Verification items for the finished model (mm, model axes). Face numbers are marked on the shaded views. A direction names the side the tool comes from. Round coordinates to 2 decimals unless told otherwise and drop trailing zeros. Write each loop counter-clockwise with the first axis right and the second up, starting at its lowest first coordinate (ties: lowest second). Pieces come first, ordered by that corner, then holes. Notation, with made-up numbers: M -27,43.5 L 22,43.5 A30 ccw 22,66.5 Z; hole C 8.25,89 d9. An arc over 180 degrees is marked long. Answer in a Markdown table with one row per item. Add a question column.
1. Go/stop test with flat-tipped pins: pin 1 Ø3 at (x, y) = (4, 75.5) entering from +Z; pin 2 Ø4 at (y, z) = (25.4, 12.7) entering from +X; pin 3 Ø4 at (x, z) = (5.5, 111) entering from +Y; pin 4 Ø4 at (x, y) = (3, 86) entering from -Z. Record where each tip stops, or that it passes through.
2. Sectioned sample at C-C on y = 95.25. Record the cut outline in (x, z).
3. Set-up check for the marked faces 1, 2 and 3: record each of +Z, -Z, +X, -X, +Y, -Y from which the full face is reachable in a straight line by a thin tool's end or side.
4. Sectioned sample at B-B on x = 2. Record the cut outline in (y, z), plus the area to 3 significant figures.
5. Sectioned sample at A-A on z = 31.75. Record the cut outline in (x, y), plus the area to 3 significant figures.
6. Material ranges on probe 1 along Y at (x, z) = (3.5, 25.4); probe 2 along Y at (x, z) = (8.25, 31.75); probe 3 along Z at (x, y) = (10, 80.5), recorded low to high.
7. Sectioned sample at D-D on z = 88.9. Record the cut outline in (x, y), plus the area to 3 significant figures.
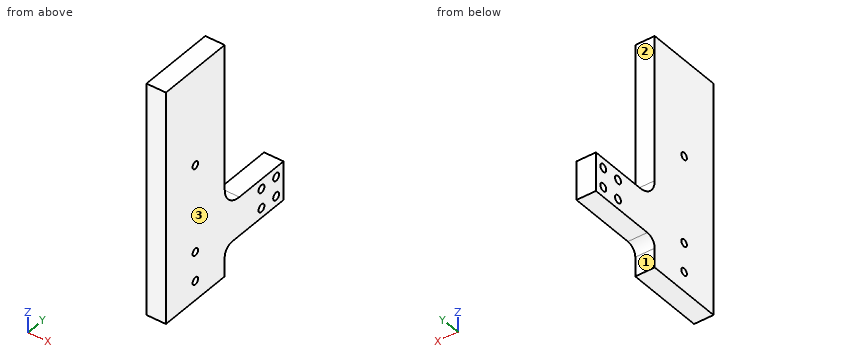
```python
from build123d import *

# Parameters (mm, degrees)
SKETCH1_R              = 2.38125
BOSS_EXTRUDE1_DEPTH    = 12.7
F_10_CLEARANCE_HOLE1_D = 5.1054
FILLET1_R              = 12.7
FILLET2_R              = 6.35


with BuildPart() as part:
    # Sketch1 → Boss-Extrude1 (new body)
    with BuildSketch(Plane(origin=(0, 0, 0), x_dir=(0, 0, -1), z_dir=(1, 0, 0))):
        Polygon((-19.05, 101.6), (-44.45, 101.6), (-44.45, 50.8), (-152.4, 50.8), (-152.4, 0), (0, 0), (0, 50.8), (-19.05, 50.8), align=None)
        with Locations((-88.9, 25.4)):
            Circle(SKETCH1_R, mode=Mode.SUBTRACT)
        with Locations((-31.75, 25.4)):
            Circle(SKETCH1_R, mode=Mode.SUBTRACT)
        with Locations((-12.7, 25.4)):
            Circle(SKETCH1_R, mode=Mode.SUBTRACT)
    extrude(amount=BOSS_EXTRUDE1_DEPTH)

    # #10 Clearance Hole1 (through all)
    with Locations(Plane(origin=(12.7, 0, 0), x_dir=(0, 0, -1), z_dir=(1, 0, 0))):
        with Locations((-38.1, 95.25), (-25.4, 95.25), (-25.4, 82.55), (-38.1, 82.55)):
            Hole(F_10_CLEARANCE_HOLE1_D / 2)

    # Fillet1
    fillet1_edges = [part.edges().sort_by_distance(p)[0] for p in [
        (6.35, 50.8, 44.45),
    ]]
    fillet(fillet1_edges, radius=FILLET1_R)

    # Fillet2
    fillet2_edges = [part.edges().sort_by_distance(p)[0] for p in [
        (6.35, 50.8, 19.05),
    ]]
    fillet(fillet2_edges, radius=FILLET2_R)


solid = part.part
```
Geometry check:
| question | item | result |
|---|---|---|
| 1 | pin 1 | stops at z = 44.45 |
| 1 | pin 2 | passes through |
| 1 | pin 3 | stops at y = 50.8 |
| 1 | pin 4 | stops at z = 19.05 |
| 2 | outline | M 0,19.05 L 12.7,19.05 L 12.7,22.85 L 0,22.85 Z; M 0,27.95 L 12.7,27.95 L 12.7,35.55 L 0,35.55 Z; M 0,40.65 L 12.7,40.65 L 12.7,44.45 L 0,44.45 Z |
| 3 | face 1 | -Z, +X, -X, +Y |
| 3 | face 2 | +Z, +X, -X, +Y |
| 3 | face 3 | +Z, -Z, +X, +Y, -Y |
| 4 | outline | M 0,0 L 50.8,0 L 50.8,12.7 A6.35 cw 57.15,19.05 L 101.6,19.05 L 101.6,44.45 L 63.5,44.45 A12.7 cw 50.8,57.15 L 50.8,152.4 L 0,152.4 Z; hole C 25.4,12.7 d4.76; hole C 25.4,31.75 d4.76; hole C 25.4,88.9 d4.76; hole C 82.55,25.4 d5.11; hole C 82.55,38.1 d5.11; hole C 95.25,25.4 d5.11; hole C 95.25,38.1 d5.11 |
| 4 | area | 8,940 mm2 |
| 5 | outline | M 0,0 L 12.7,0 L 12.7,23.02 L 0,23.02 Z; M 0,27.78 L 12.7,27.78 L 12.7,101.6 L 0,101.6 Z |
| 5 | area | 1,230 mm2 |
| 6 | probe 1 | y = 0 to 80, 85.1 to 92.7, 97.8 to 101.6 |
| 6 | probe 2 | y = 0 to 23.02, 27.78 to 101.6 |
| 6 | probe 3 | z = 19.05 to 23.88, 26.92 to 36.58, 39.62 to 44.45 |
| 7 | outline | M 0,0 L 12.7,0 L 12.7,23.02 L 0,23.02 Z; M 0,27.78 L 12.7,27.78 L 12.7,50.8 L 0,50.8 Z |
| 7 | area | 585 mm2 |
